Design review of the part built by this model. Coordinates are the model's own, in mm. Coordinates: 2 decimals unless noted, no trailing zeros. Answer in a Markdown table with one row per item. Add a question column.
(1) We need section A-A, the plane x = -112.5. Give the number of separate pieces and of enclosed holes in the cut face, plus the area to 3 significant figures.
(2) The part is to be moulded in two halves that separate along X. For faces 1 (the face through (-26.836, 1.521, -47.976)), 2 (the face through (19.9, 1.52, 137.67)), say which applies: released by +X, released by -X, zero draft, split by the parting line, or undercut.
(3) Clearance check with a flat-ended pin moving along its axis: pin 1 (24 mm diameter, centred on x = 157.5, z = 157.5, fed in from +Y). State where the tip first meets the part, or that it passes through.
from build123d import *

# Parameters (mm, degrees)
SKETCH1_W            = 395
SKETCH1_H            = 395
SKETCH1_R            = 2.55
BOSS_EXTRUDE1_DEPTH  = 3
FILLET1_R            = 15
SKETCH2_R            = 20
CUT_EXTRUDE1_DEPTH   = 4
LPATTERN1_COUNT      = 8
LPATTERN1_PITCH      = 45
LPATTERN1_COUNT_DIR2 = 8
LPATTERN1_PITCH_DIR2 = 45


with BuildPart() as part:
    # Sketch1 → Boss-Extrude1 (new body)
    with BuildSketch(Plane(origin=(0, 0, 0), x_dir=(1, 0, 0), z_dir=(0, 1, 0))):
        Rectangle(SKETCH1_W, SKETCH1_H)
        with Locations((-182.5, 182.5)):
            Circle(SKETCH1_R, mode=Mode.SUBTRACT)
        with Locations((182.5, 182.5)):
            Circle(SKETCH1_R, mode=Mode.SUBTRACT)
        with Locations((182.5, -182.5)):
            Circle(SKETCH1_R, mode=Mode.SUBTRACT)
        with Locations((-182.5, -182.5)):
            Circle(SKETCH1_R, mode=Mode.SUBTRACT)
    extrude(amount=BOSS_EXTRUDE1_DEPTH)

    # Fillet1
    fillet1_edges = [part.edges().sort_by_distance(p)[0] for p in [
        (197.5, 1.5, 197.5),
        (-197.5, 1.5, 197.5),
        (-197.5, 1.5, -197.5),
        (197.5, 1.5, -197.5),
    ]]
    fillet(fillet1_edges, radius=FILLET1_R)

    # Sketch2 → Cut-Extrude1 (cut, through all)
    with BuildSketch(Plane(origin=(0, 3, 0), x_dir=(1, 0, 0), z_dir=(0, 1, 0))):
        with Locations((-157.5, -157.5)):
            Circle(SKETCH2_R)
    cut_extrude1 = extrude(amount=-CUT_EXTRUDE1_DEPTH, mode=Mode.SUBTRACT)

    # LPattern1: Cut-Extrude1 8 × 8
    with Locations(*[(j * LPATTERN1_PITCH_DIR2, 0, -i * LPATTERN1_PITCH) for i in range(LPATTERN1_COUNT) for j in range(LPATTERN1_COUNT_DIR2) if (i, j) != (0, 0)]):
        add(cut_extrude1, mode=Mode.SUBTRACT)


solid = part.part
Responses:
| question | item | result |
|---|---|---|
| 1 | separate pieces | 9 |
| 1 | enclosed holes | 0 |
| 1 | area | 225 mm2 |
| 2 | face 1 | undercut |
| 2 | face 2 | undercut |
| 3 | pin 1 | passes through |
